```python
from build123d import *

# Parameters (mm, degrees)
SKETCH1_W                     = 40
SKETCH1_H                     = 40
BOSS_EXTRUDE1_DEPTH           = 1
SKETCH2_R                     = 7.5
SKETCH2_R_2                   = 6.5
BOSS_EXTRUDE2_DEPTH           = 2
M3_CLEARANCE_HOLE1_AT_2_COUNT = 2
M3_CLEARANCE_HOLE1_AT_2_PITCH = 34
M3_CLEARANCE_HOLE1_AT_3_COUNT = 2
M3_CLEARANCE_HOLE1_AT_3_PITCH = 48.083261121
M3_CLEARANCE_HOLE1_AT_4_COUNT = 2
M3_CLEARANCE_HOLE1_AT_4_PITCH = 34


with BuildPart() as part:
    # Sketch1 → Boss-Extrude1 (new body)
    with BuildSketch(Plane(origin=(0, 0, 0), x_dir=(1, 0, 0), z_dir=(0, 1, 0))):
        with Locations((20, 20)):
            Rectangle(SKETCH1_W, SKETCH1_H)
    extrude(amount=BOSS_EXTRUDE1_DEPTH)

    # Sketch2 → Boss-Extrude2 (add)
    with BuildSketch(Plane(origin=(0, 1, 0), x_dir=(1, 0, 0), z_dir=(0, 1, 0))):
        with Locations(Location((20, 20, 0), (0, 0, 90))):
            Circle(SKETCH2_R)
        with Locations(Location((20, 20, 0), (0, 0, 270))):
            Circle(SKETCH2_R_2, mode=Mode.SUBTRACT)
    extrude(amount=BOSS_EXTRUDE2_DEPTH)

    # Sketch4 → M3 Clearance Hole1 (revolve, cut)
    with BuildSketch(Plane(origin=(3, 1, -3), x_dir=(0, 0, 1), z_dir=(1, 0, 0))):
        Polygon((0, 0), (0, 1), (1.7, 1), (1.7, 0.025), (1.725, 0), align=None)
    m3_clearance_hole1 = revolve(axis=Axis((3, 7.35, -3), (0, -1, 0)), mode=Mode.SUBTRACT)

    # M3 Clearance Hole1 at 2: M3 Clearance Hole1 ×2
    with Locations(*[(0, 0, -i * M3_CLEARANCE_HOLE1_AT_2_PITCH) for i in range(1, M3_CLEARANCE_HOLE1_AT_2_COUNT)]):
        add(m3_clearance_hole1, mode=Mode.SUBTRACT)

    # M3 Clearance Hole1 at 3: M3 Clearance Hole1 ×2
    with Locations(*[Vector(0.7071067811865477, 0, -0.7071067811865474) * (i * M3_CLEARANCE_HOLE1_AT_3_PITCH) for i in range(1, M3_CLEARANCE_HOLE1_AT_3_COUNT)]):
        add(m3_clearance_hole1, mode=Mode.SUBTRACT)

    # M3 Clearance Hole1 at 4: M3 Clearance Hole1 ×2
    with Locations(*[(i * M3_CLEARANCE_HOLE1_AT_4_PITCH, 0, 0) for i in range(1, M3_CLEARANCE_HOLE1_AT_4_COUNT)]):
        add(m3_clearance_hole1, mode=Mode.SUBTRACT)


solid = part.part
```
The listing builds one solid part. Answer for the finished solid, in the listing's coordinates (mm). A direction names the side the tool comes from. Give positions to 0.01 mm unless a question says otherwise; leave off trailing zeros. Order: outer loops, then holes, each group sorted by start corner. A loop starts at its lowest first (then second) coordinate and runs counter-clockwise, first axis right, second up. Notation, with made-up numbers: (-10, 8.5) -> (36, 8.5) arc R13 ccw to (36, 25.5) -> close; hole circle Ø7 at (-27, 66.5). An arc over 180 degrees is marked (long way). One line per item, written item: value.
1) Find section A-A, the plane z = -3. Determine the outline of the cut face in (x, y) (3 decimals), plus the area to 3 significant figures.
Reported:
outline: (0, 0) -> (1.3, 0) -> (1.3, 0.975) -> (1.275, 1) -> (0, 1) -> close; (4.7, 0) -> (35.3, 0) -> (35.3, 0.975) -> (35.275, 1) -> (4.725, 1) -> (4.7, 0.975) -> close; (38.7, 0) -> (40, 0) -> (40, 1) -> (38.725, 1) -> (38.7, 0.975) -> close
area: 33.2 mm^2
2) A tool of negligible diameter and unlimited length cuts with its end or side. For faces 1 (the cylindrical face through (19.67, 1.986, -12.507)), 2 (the cylindrical face through (38.5, 0.5, -2.2)), from which of +Z, -Z, +X, -X, +Y, -Y can it reach the whole face along a straight path? Write none if from no direction.
Reported:
face 1: +Y
face 2: +Y, -Y
3) Find section B-B, the plane x = 3. Determine the outline of the cut face in (y, z) (3 decimals).
Reported:
outline: (0, -40) -> (1, -40) -> (1, -38.725) -> (0.975, -38.7) -> (0, -38.7) -> close; (0, -35.3) -> (0.975, -35.3) -> (1, -35.275) -> (1, -4.725) -> (0.975, -4.7) -> (0, -4.7) -> close; (0, -1.3) -> (0.975, -1.3) -> (1, -1.275) -> (1, 0) -> (0, 0) -> close
4) Find the intervals of material crossed by line 1 (X direction, y = 0.6, z = -37); line 2 (Z direction, x = 3, y = 0.7); line 3 (X direction, y = 1.1, z = -20), in increasing order.
Reported:
line 1: x = 0 to 1.3, 4.7 to 35.3, 38.7 to 40
line 2: z = -40 to -38.7, -35.3 to -4.7, -1.3 to 0
line 3: x = 12.5 to 13.5, 26.5 to 27.5
5) Find section D-D, the plane y = 2.35. Determine the outline of the cut face in (x, z).
Reported:
outline: circle Ø15 at (20, -20); hole circle Ø13 at (20, -20)
6) Find section C-C, the plane x = 20. Determine the outline of the cut face in (y, z), plus the area to 3 significant figures.
Reported:
outline: (0, -40) -> (1, -40) -> (1, -27.5) -> (3, -27.5) -> (3, -26.5) -> (1, -26.5) -> (1, -13.5) -> (3, -13.5) -> (3, -12.5) -> (1, -12.5) -> (1, 0) -> (0, 0) -> close
area: 44.0 mm^2
7) Determine the mould class of faces 3 (the flat face through (20, 1, -20)), 4 (the flat face through (17, 3, -14)), 5 (the flat face through (0, 0.5, -19.7)), 6 (the cylindrical face through (1.85, 0.49, -38.25)) for opening direction X: pulls with the +X half, pulls with the -X half, needs draft (parallel to the pull), parting line crosses it, or undercut.
Reported:
face 3: undercut
face 4: needs draft
face 5: pulls with the -X half
face 6: undercut
8) Flat-ended cylindrical pins translate along their axes: P1, Ø15, axis at x = 20, z = -20, coming from the +Y side; P2, Ø2, axis at x = 17.5, z = -30, coming from the +Y side; P3, Ø2.5, axis at x = 3, z = -3, coming from the +Y side. Find the tip coordinate at first contact, or state that the pin passes through.
Reported:
P1: stops at y = 3
P2: stops at y = 1
P3: passes through
